Design review of the part built by this model. Coordinates are the model's own, in mm. Round coordinates to 2 decimals unless told otherwise and drop trailing zeros. Loops run counter-clockwise (first coordinate to the right, second up) from the corner with the lowest first, then second, coordinate; pieces in that order, holes last. Notation, with made-up numbers: (3.25, -35) - (14.25, -35) arc R18 ccw to (14.25, -28) - close; hole circle Ø11 at (64.5, 69). An arc over 180 degrees is marked (long way). Answer as CSV lines item,"result". Start each with the question number.
(1) Wall thickness on L1, parallel to Y at x = -5, z = 2.7 (3 decimals); L2, parallel to X at y = 13, z = 2.15; L3, parallel to X at y = 20, z = 1.8: over which ranges is each line inside the solid? List them lowest first.
(2) Consider section C-C (y = 38). Give the boundary of the cut face in (x, z).
(3) Consider section B-B (y = 17.5). Give the boundary of the cut face in (x, z).
(4) Consider section A-A (x = 42). Give the boundary of the cut face in (y, z).
(5) Consider section D-D (x = -46.45). Give the boundary of the cut face in (y, z) (3 decimals).
(6) For P1, Ø2.5, axis at x = -73, z = 1.5, coming from the -Y side; P2, Ø1.5, axis at x = 73, z = 2.5, coming from the +Y side; P3, Ø1.5, axis at y = 38.5, z = 2, coming from the +X side, all flat-tipped, find the tip position at first contact; note any pin that passes through.
from build123d import *

# Parameters (mm, degrees)
BOSS_EXTRUDE1_DEPTH = 5
SKETCH2_R           = 1.25
SKETCH2_W           = 64.4
SKETCH2_H           = 14.51
SKETCH2_W_2         = 20
SKETCH2_H_2         = 20
CUT_EXTRUDE1_DEPTH  = 5
SKETCH3_R           = 2.5
SKETCH3_R_2         = 1.5
SKETCH3_W           = 46.6
SKETCH3_H           = 9
SKETCH3_W_2         = 15
SKETCH3_H_2         = 8
SKETCH3_H_3         = 11
SKETCH3_W_3         = 50
SKETCH3_H_4         = 5
CUT_EXTRUDE2_DEPTH  = 10
FILLET1_R           = 0.5


with BuildPart() as part:
    # Sketch1 → Boss-Extrude1 (new body)
    with BuildSketch(Plane.XY):
        Polygon((-75, -15), (-70, -15), (-70, -40), (70, -40), (70, -15), (75, -15), (75, 15), (70, 15), (70, 45), (-70, 45), (-70, 15), (-75, 15), align=None)
    extrude(amount=BOSS_EXTRUDE1_DEPTH)

    # Sketch2 → Cut-Extrude1 (cut)
    with BuildSketch(Plane.XY.offset(5)):
        with Locations((-57.5, 30.5)):
            Circle(SKETCH2_R)
        with Locations((17.5, 30.5)):
            Circle(SKETCH2_R)
        with Locations((17.5, -0.5)):
            Circle(SKETCH2_R)
        with Locations((-57.5, -0.5)):
            Circle(SKETCH2_R)
        with Locations((27.6, 32.132337083)):
            Circle(SKETCH2_R)
        with Locations((52.4, 32.132337083)):
            Circle(SKETCH2_R)
        with Locations((22.75, -5.367662917)):
            Circle(SKETCH2_R)
        with Locations((57.25, -5.367662917)):
            Circle(SKETCH2_R)
        with Locations((-20, 15)):
            Rectangle(SKETCH2_W, SKETCH2_H)
        with Locations((40, 15)):
            Rectangle(SKETCH2_W_2, SKETCH2_H_2)
    extrude(amount=-CUT_EXTRUDE1_DEPTH, mode=Mode.SUBTRACT)

    # Sketch3 → Cut-Extrude2 (cut)
    with BuildSketch(Plane.XY.offset(5)):
        with Locations((-54.45, -11)):
            Circle(SKETCH3_R)
        with Locations((-46.45, -11)):
            Circle(SKETCH3_R)
        with Locations((-37.4, -6.5)):
            Circle(SKETCH3_R)
        with Locations((-28.45, -11)):
            Circle(SKETCH3_R)
        with Locations((-20.45, -11)):
            Circle(SKETCH3_R)
        with Locations((72.5, 0)):
            Circle(SKETCH3_R_2)
        with Locations((-72.5, 0)):
            Circle(SKETCH3_R_2)
        with Locations((-37.4, -13.5)):
            Circle(SKETCH3_R)
        with Locations((-3.8, 37.255)):
            Rectangle(SKETCH3_W, SKETCH3_H)
        with Locations((-9.3, -12.755)):
            Rectangle(SKETCH3_W_2, SKETCH3_H_2)
        with Locations((8.7, -8.755)):
            Rectangle(SKETCH3_W_2, SKETCH3_H_3)
        with Locations((-20, -32.5)):
            Rectangle(SKETCH3_W_3, SKETCH3_H_4)
    extrude(amount=-CUT_EXTRUDE2_DEPTH, mode=Mode.SUBTRACT)

    # Fillet1
    fillet1_edges = [part.edges().sort_by_distance(p)[0] for p in [
        (16.2, -3.255, 2.5),
        (16.2, -14.255, 2.5),
        (1.2, -14.255, 2.5),
        (1.2, -3.255, 2.5),
        (-1.8, -8.755, 2.5),
        (-1.8, -16.755, 2.5),
        (-16.8, -16.755, 2.5),
        (-16.8, -8.755, 2.5),
    ]]
    fillet(fillet1_edges, radius=FILLET1_R)


solid = part.part
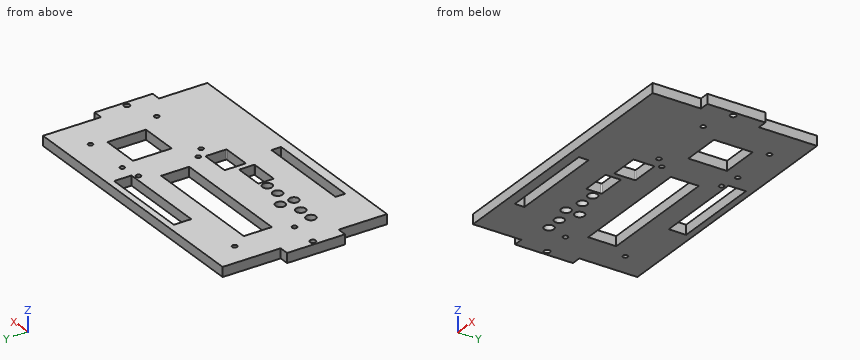
Determined:
1,L1,"y = -40 to -35, -30 to -16.755, -8.755 to 7.745, 22.255 to 32.755, 41.755 to 45"
1,L2,"x = -75 to -52.2, 12.2 to 30, 50 to 75"
1,L3,"x = -70 to -52.2, 12.2 to 30, 50 to 70"
2,outline,"(-70, 0) - (-27.1, 0) - (-27.1, 5) - (-70, 5) - close; (19.5, 0) - (70, 0) - (70, 5) - (19.5, 5) - close"
3,outline,"(-70, 0) - (-52.2, 0) - (-52.2, 5) - (-70, 5) - close; (12.2, 0) - (30, 0) - (30, 5) - (12.2, 5) - close; (50, 0) - (70, 0) - (70, 5) - (50, 5) - close"
4,outline,"(-40, 0) - (5, 0) - (5, 5) - (-40, 5) - close; (25, 0) - (45, 0) - (45, 5) - (25, 5) - close"
5,outline,"(-40, 0) - (-13.5, 0) - (-13.5, 5) - (-40, 5) - close; (-8.5, 0) - (7.745, 0) - (7.745, 5) - (-8.5, 5) - close; (22.255, 0) - (45, 0) - (45, 5) - (22.255, 5) - close"
6,P1,"stops at y = -15"
6,P2,"stops at y = 15"
6,P3,"stops at x = 70"
